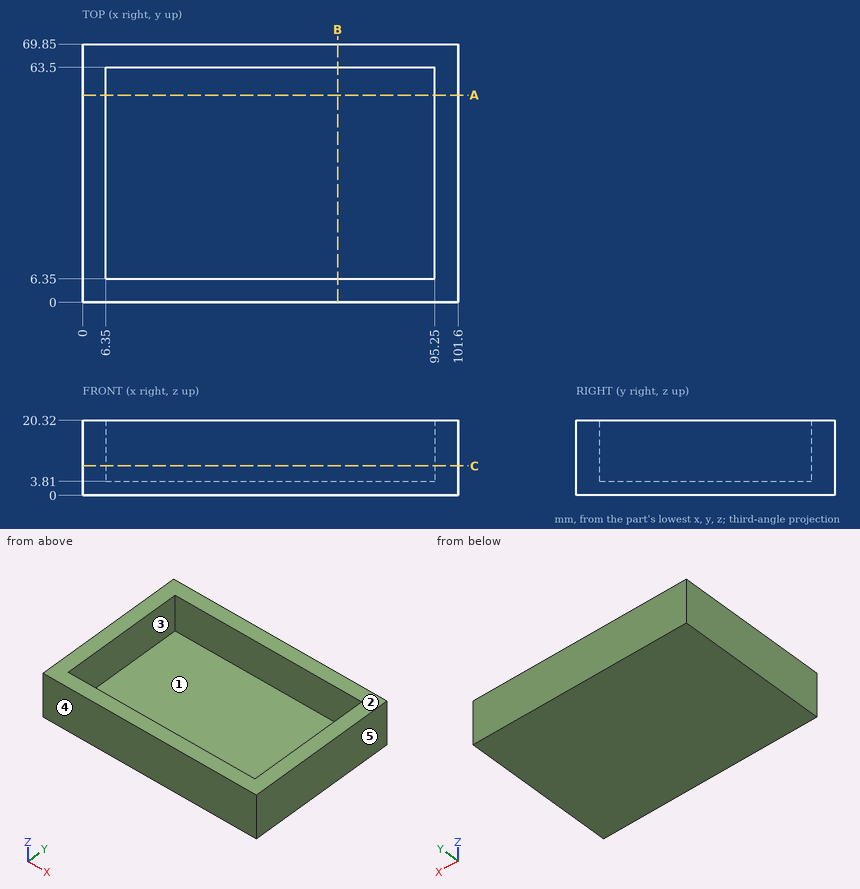
Answer from the drawing. Dimensions are ordinates in mm from the lowest x, y and z of the part. A direction names the side the tool comes from. Give positions to 0.01 mm unless a question says otherwise; leave off trailing zeros. Order: outer loops, then holes, each group sorted by start corner. A loop starts at its lowest first (then second) coordinate and runs counter-clockwise, first axis right, second up. Notation, with made-up numbers: (16.5, -35.5) -> (65.5, -35.5) arc R10 ccw to (65.5, -21.5) -> close; hole circle Ø6 at (9, 79.5). An arc over 180 degrees is marked (long way). One line per item, written item: value.
Item 1: Find section C-C, the plane z = 8. Give the vertices of the cut face in (x, y).
Answer sheet:
outline: (0, 0) -> (101.6, 0) -> (101.6, 69.85) -> (0, 69.85) -> close; hole (6.35, 6.35) -> (95.25, 6.35) -> (95.25, 63.5) -> (6.35, 63.5) -> close
Item 2: Find section A-A, the plane y = 56. Give the vertices of the cut face in (x, z).
Answer sheet:
outline: (0, 0) -> (101.6, 0) -> (101.6, 20.32) -> (95.25, 20.32) -> (95.25, 3.81) -> (6.35, 3.81) -> (6.35, 20.32) -> (0, 20.32) -> close
Item 3: A tool of negligible diameter and unlimited length cuts with its end or side. For the marked faces 1 and 2, from which of +Z, -Z, +X, -X, +Y, -Y can it reach the whole face along a straight path? Write none if from no direction.
Answer sheet:
face 1: +Z
face 2: +Z, +X, -X, +Y, -Y
Item 4: Determine the mould class of the marked faces 3, 4 and 5 for opening direction X: released by +X, released by -X, zero draft, split by the parting line, or undercut.
Answer sheet:
face 3: undercut
face 4: zero draft
face 5: released by +X
Item 5: Straight lines are drawn through the part: probe 1 along Y at (x, z) = (57, 16.75); probe 2 along X at (y, z) = (21, 16); probe 3 along Z at (x, y) = (55, 7). For each, find the intervals that lie inside material, in ascending order.
Answer sheet:
probe 1: 0 to 6.35, 63.5 to 69.85
probe 2: 0 to 6.35, 95.25 to 101.6
probe 3: 0 to 3.81
Item 6: Find section B-B, the plane x = 69. Give the vertices of the cut face in (y, z), plus the area to 3 significant figures.
Answer sheet:
outline: (0, 0) -> (69.85, 0) -> (69.85, 20.32) -> (63.5, 20.32) -> (63.5, 3.81) -> (6.35, 3.81) -> (6.35, 20.32) -> (0, 20.32) -> close
area: 476 mm²
